Check sheet for the drawn part. Datum: minimum x, y, z corner. Units: mm. A direction names the side the tool comes from. Round coordinates to 2 decimals unless told otherwise and drop trailing zeros. Order: outer loops, then holes, each group sorted by start corner. A loop starts at its lowest first (then second) coordinate and runs counter-clockwise, first axis right, second up. Notation, with made-up numbers: (-19.5, 57.5) -> (37.5, 57.5) arc R16 cw to (37.5, 71.5) -> close; hole circle Ø6 at (-10, -37). An arc over 180 degrees is marked (long way). Use CSV: the item, a comma, the result in double quotes.
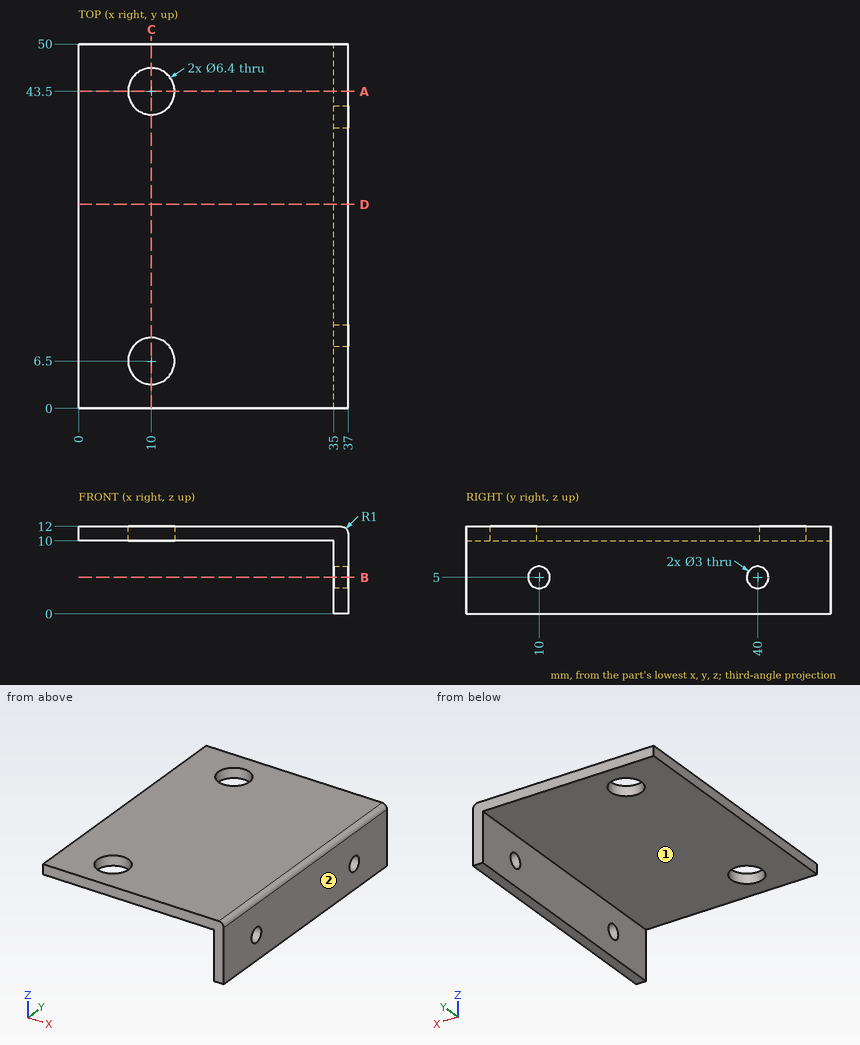
Q1. Sectioned sample at D-D, the plane y = 28. Enter the section's corners in (x, z).
Result sheet:
outline,"(0, 10) -> (35, 10) -> (35, 0) -> (37, 0) -> (37, 11) arc R1 ccw to (36, 12) -> (0, 12) -> close"
Q2. Sectioned sample at A-A, the plane y = 43.5. Enter the section's corners in (x, z), then the cut area to 3 significant figures.
Result sheet:
outline,"(0, 10) -> (6.8, 10) -> (6.8, 12) -> (0, 12) -> close; (13.2, 10) -> (35, 10) -> (35, 0) -> (37, 0) -> (37, 11) arc R1 ccw to (36, 12) -> (13.2, 12) -> close"
area,"81.0 mm^2"
Q3. Scan lines: L1, parallel to Y at x = 10, z = 11; L2, parallel to Y at x = 35.5, z = 5; L3, parallel to X at y = 14, z = 0.5. Record each from-to range of solid material in increasing order.
Result sheet:
L1,"y = 0 to 3.3, 9.7 to 40.3, 46.7 to 50"
L2,"y = 0 to 8.5, 11.5 to 38.5, 41.5 to 50"
L3,"x = 35 to 37"
Q4. Sectioned sample at B-B, the plane z = 5. Enter the section's corners in (x, y).
Result sheet:
outline,"(35, 0) -> (37, 0) -> (37, 8.5) -> (35, 8.5) -> close; (35, 11.5) -> (37, 11.5) -> (37, 38.5) -> (35, 38.5) -> close; (35, 41.5) -> (37, 41.5) -> (37, 50) -> (35, 50) -> close"
Q5. Go/stop test with flat-tipped pins: pin 1 (8.5 mm diameter, centred on x = 10, y = 6.5, fed in from -Z); pin 2 (3 mm diameter, centred on y = 36.5, z = 4.5, fed in from -X); pin 3 (1.8 mm diameter, centred on y = 40, z = 5, fed in from -X). Record where each tip stops, or that it passes through.
Result sheet:
pin 1,"stops at z = 10"
pin 2,"stops at x = 35"
pin 3,"passes through"
Q6. Sectioned sample at C-C, the plane x = 10. Enter the section's corners in (y, z), then the cut area to 3 significant figures.
Result sheet:
outline,"(0, 10) -> (3.3, 10) -> (3.3, 12) -> (0, 12) -> close; (9.7, 10) -> (40.3, 10) -> (40.3, 12) -> (9.7, 12) -> close; (46.7, 10) -> (50, 10) -> (50, 12) -> (46.7, 12) -> close"
area,"74.4 mm^2"
Q7. Access from +Z, -Z, +X, -X, +Y, -Y to the whole of each face (thin tool, end or side, straight path). Record for the marked faces 1 and 2.
Result sheet:
face 1,"-Z, -X, +Y, -Y"
face 2,"+Z, -Z, +X, +Y, -Y"
